Verification items for this drawing (mm, ordinates from the low corner). A direction names the side the tool comes from. Give positions to 0.01 mm unless a question says otherwise; leave off trailing zeros. Order: outer loops, then holes, each group sorted by start corner. A loop starts at its lowest first (then second) coordinate and runs counter-clockwise, first axis right, second up.
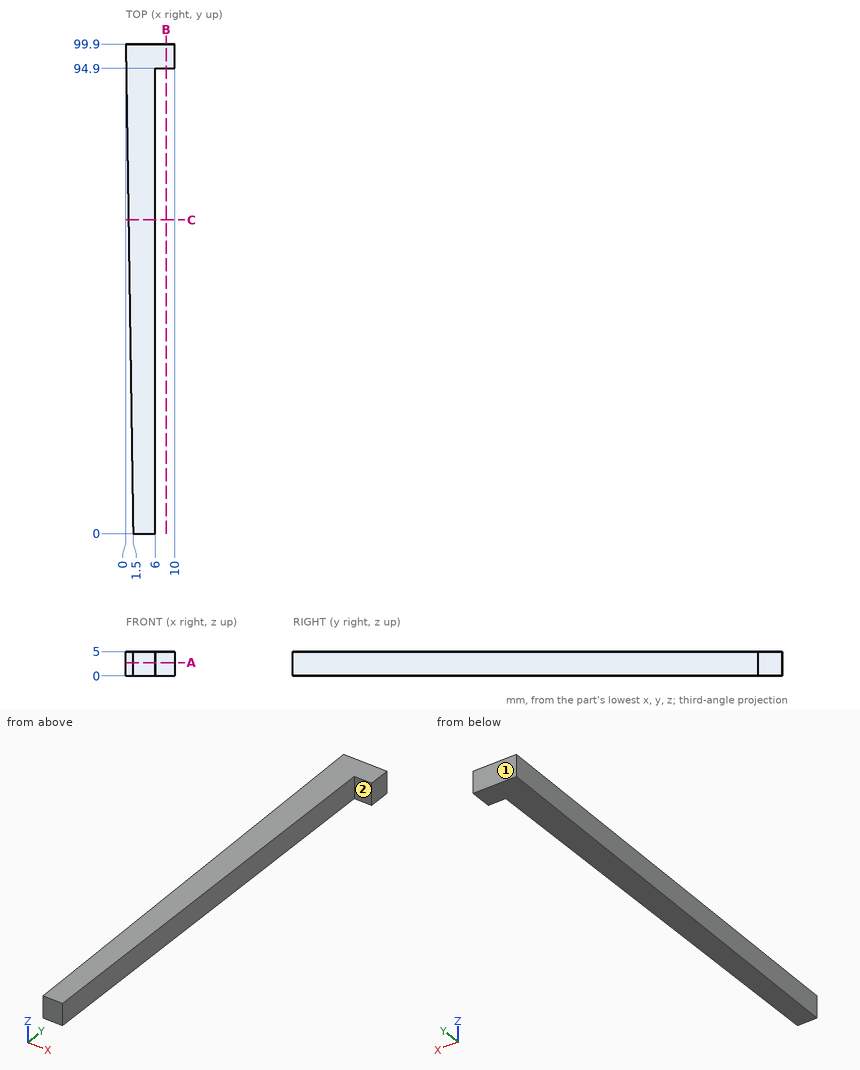
Q1. Access from +Z, -Z, +X, -X, +Y, -Y to the whole of each face (thin tool, end or side, straight path). Record for the marked faces 1 and 2.
Q2. Thickness scan on L1, parallel to Y at x = 7, z = 2.45; L2, parallel to X at y = 48, z = 3.45; L3, parallel to X at y = 93, z = 0.25. Record the ranges inside material, lowest first.
Q3. Cross-section at B-B, the plane x = 8.25. Record the boundary of the cut face in (y, z), and give its area (3 significant figures).
Q4. Cross-section at A-A, the plane z = 2.75. Record the boundary of the cut face in (x, y).
Q5. Cross-section at C-C, the plane y = 64. Record the boundary of the cut face in (x, z).
Q6. Gauge pin test, flat ends, axial feed: P1, Ø1.2, axis at x = 9, z = 2.5, coming from the -Y side; P2, Ø3, axis at y = 55.5, z = 4.5, coming from the -X side; P3, Ø1.5, axis at y = 71.5, z = 2, coming from the -X side. Record the tip position at first contact, or that the pin passes through.
Answers follow:
1. face 1: +Z, -Z, +X, -X, +Y
1. face 2: +Z, -Z, +X, -Y
2. L1: y = 94.9 to 99.9
2. L2: x = 0.78 to 6
2. L3: x = 0.1 to 6
3. outline: (94.9, 0) - (99.9, 0) - (99.9, 5) - (94.9, 5) - close
3. area: 25.0 mm2
4. outline: (0, 99.9) - (1.5, 0) - (6, 0) - (6, 94.9) - (10, 94.9) - (10, 99.9) - close
5. outline: (0.54, 0) - (6, 0) - (6, 5) - (0.54, 5) - close
6. P1: stops at y = 94.9
6. P2: stops at x = 0.64
6. P3: stops at x = 0.42
